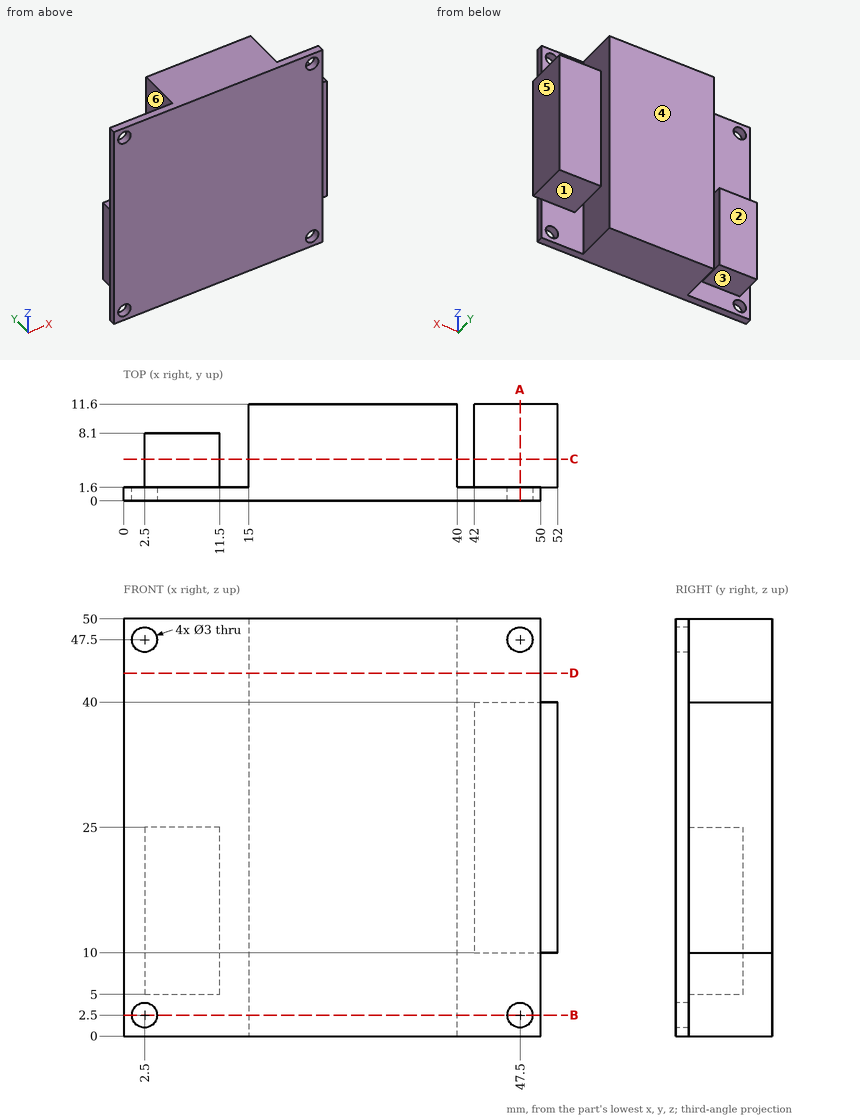
Study the drawing (mm; zero at the part's minimum x, y, z) and answer. A direction names the side the tool comes from. Round coordinates to 2 decimals unless told otherwise and drop trailing zeros. Order: outer loops, then holes, each group sorted by start corner. A loop starts at its lowest first (then second) coordinate and runs counter-clockwise, first axis right, second up. Notation, with made-up numbers: (12.25, 89) -> (60.25, 89) arc R20 cw to (60.25, 93) -> close; hole circle Ø9 at (53, 66.5). An arc over 180 degrees is marked (long way). Answer as CSV lines item,"result". Start each with the question number.
(1) A tool of negligible diameter and unlimited length cuts with its end or side. For the marked faces 1, 2 and 3, from which of +Z, -Z, +X, -X, +Y, -Y can it reach the whole face along a straight path? Write none if from no direction.
(2) The part is cut by section A-A (x = 47.5). Determine the outline of the cut face in (y, z).
(3) Flat-ended cylindrical pins translate along their axes: pin 1 Ø2 at (x, z) = (13.5, 28.5) entering from +Y; pin 2 Ø3 at (y, z) = (8, 25.5) entering from -X; pin 3 Ø2.5 at (x, z) = (47.5, 47.5) entering from -Y; pin 4 Ø7.5 at (x, z) = (11, 17) entering from +Y. Find the tip coordinate at first contact, or state that the pin passes through.
(4) For a pull along X with two mould halves and no side action, classify the marked faces 4, 5 and 6 as +X half, -X half, draft (parallel to the pull), parting line (faces both ways), or undercut.
(5) The part is cut by section B-B (z = 2.5). Determine the outline of the cut face in (x, y).
(6) Find the intervals of material crossed by probe 1 along Z at (x, y) = (2.5, 1.05); probe 2 along X at (y, z) = (7, 14.5); probe 3 along X at (y, z) = (11.25, 16), in increasing order. Write a range as from..to.
(7) The part is cut by section D-D (z = 43.5). Determine the outline of the cut face in (x, y).
(8) The part is cut by section C-C (y = 5). Determine the outline of the cut face in (x, z), then the cut area to 3 significant figures.
Evaluation:
1,face 1,"-Z, +X, +Y"
1,face 2,"+Z, -Z, -X, +Y"
1,face 3,"-Z, -X, +Y"
2,outline,"(0, 0) -> (1.6, 0) -> (1.6, 1) -> (0, 1) -> close; (0, 4) -> (1.6, 4) -> (1.6, 10) -> (11.6, 10) -> (11.6, 40) -> (1.6, 40) -> (1.6, 46) -> (0, 46) -> close; (0, 49) -> (1.6, 49) -> (1.6, 50) -> (0, 50) -> close"
3,pin 1,"y = 1.6"
3,pin 2,"x = 2.5"
3,pin 3,"through"
3,pin 4,"y = 8.1"
4,face 4,"draft"
4,face 5,"+X half"
4,face 6,"undercut"
5,outline,"(0, 0) -> (1, 0) -> (1, 1.6) -> (0, 1.6) -> close; (4, 0) -> (46, 0) -> (46, 1.6) -> (40, 1.6) -> (40, 11.6) -> (15, 11.6) -> (15, 1.6) -> (4, 1.6) -> close; (49, 0) -> (50, 0) -> (50, 1.6) -> (49, 1.6) -> close"
6,probe 1,"0..1, 4..46, 49..50"
6,probe 2,"2.5..11.5, 15..40, 42..52"
6,probe 3,"15..40, 42..52"
7,outline,"(0, 0) -> (50, 0) -> (50, 1.6) -> (40, 1.6) -> (40, 11.6) -> (15, 11.6) -> (15, 1.6) -> (0, 1.6) -> close"
8,outline,"(2.5, 5) -> (11.5, 5) -> (11.5, 25) -> (2.5, 25) -> close; (15, 0) -> (40, 0) -> (40, 50) -> (15, 50) -> close; (42, 10) -> (52, 10) -> (52, 40) -> (42, 40) -> close"
8,area,"1,730 mm²"
